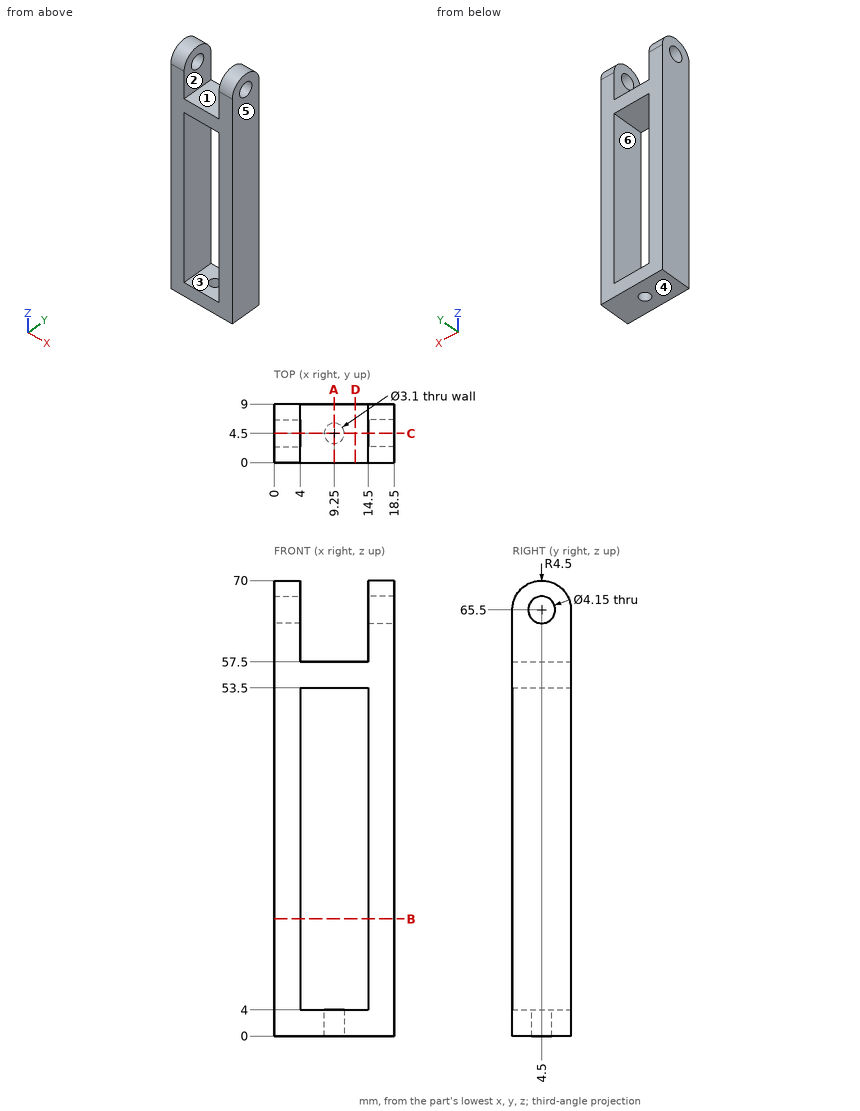
The drawing under review shows one solid part. Ordinate dimensions are in mm from its lowest x, y, z. A direction names the side the tool comes from. Give positions to 0.01 mm unless a question says otherwise; leave off trailing zeros. Order: outer loops, then holes, each group sorted by start corner. A loop starts at its lowest first (then second) coordinate and runs counter-clockwise, first axis right, second up. Notation, with made-up numbers: M 83.5,46 L 105.5,46 A20 cw 105.5,58 Z; hole C 26.25,-16 d3. An arc over 180 degrees is marked long. One line per question, with ' | ' between items. Start each with the question number.
Q1. We need section B-B (z = 18). Write out the cut boundary in (x, y).
Q2. We need section C-C (y = 4.5). Write out the cut boundary in (x, z) (3 decimals).
Q3. For L1, parallel to X at y = 2.5, z = 33; L2, parallel to Y at x = 17.2, z = 65.5 (3 decimals); L3, parallel to Z at x = 13.5, y = 2.5, list the stretches that pass through material, from the lowest coordinate up. Write a range as [from, to].
Q4. The part is to be moulded in two halves that separate along Z. For the marked faces 1, 2, 3 and 4, say which applies: +Z half, -Z half, draft (parallel to the pull), parting line (faces both ways), or undercut.
Q5. We need section D-D (x = 12.5). Write out the cut boundary in (y, z), plus the area to 3 significant figures.
Q6. Machinability: for the marked faces 5 and 6, which of the approach directions +Z, -Z, +X, -X, +Y, -Y give a long, thin tool a straight path to every point of the face, cutting with its end or side? Answer none if there is none.
Q7. We need section A-A (x = 9.25). Write out the cut boundary in (y, z).
Q8. For pin 1 Ø1 at (x, y) = (15.5, 1.5) entering from +Z; pin 2 Ø4 at (x, y) = (9.25, 4.5) entering from +Z; pin 3 Ø2 at (x, z) = (12, 14.5) entering from +Y, all flat-tipped, find the tip position at first contact; note any pin that passes through.
Returned:
1) outline: M 0,0 L 4,0 L 4,9 L 0,9 Z; M 14.5,0 L 18.5,0 L 18.5,9 L 14.5,9 Z
2) outline: M 0,0 L 7.7,0 L 7.7,4 L 4,4 L 4,53.5 L 14.5,53.5 L 14.5,4 L 10.8,4 L 10.8,0 L 18.5,0 L 18.5,63.425 L 14.5,63.425 L 14.5,57.5 L 4,57.5 L 4,63.425 L 0,63.425 Z; M 0,67.575 L 4,67.575 L 4,70 L 0,70 Z; M 14.5,67.575 L 18.5,67.575 L 18.5,70 L 14.5,70 Z
3) L1: [0, 4], [14.5, 18.5] | L2: [0, 2.425], [6.575, 9] | L3: [0, 4], [53.5, 57.5]
4) face 1: +Z half | face 2: draft | face 3: undercut | face 4: -Z half
5) outline: M 0,0 L 9,0 L 9,4 L 0,4 Z; M 0,53.5 L 9,53.5 L 9,57.5 L 0,57.5 Z | area: 72.0 mm2
6) face 5: +Z, -Z, +X, +Y, -Y | face 6: +Y, -Y
7) outline: M 0,0 L 2.95,0 L 2.95,4 L 0,4 Z; M 0,53.5 L 9,53.5 L 9,57.5 L 0,57.5 Z; M 6.05,0 L 9,0 L 9,4 L 6.05,4 Z
8) pin 1: z = 69.24 | pin 2: z = 57.5 | pin 3: through
